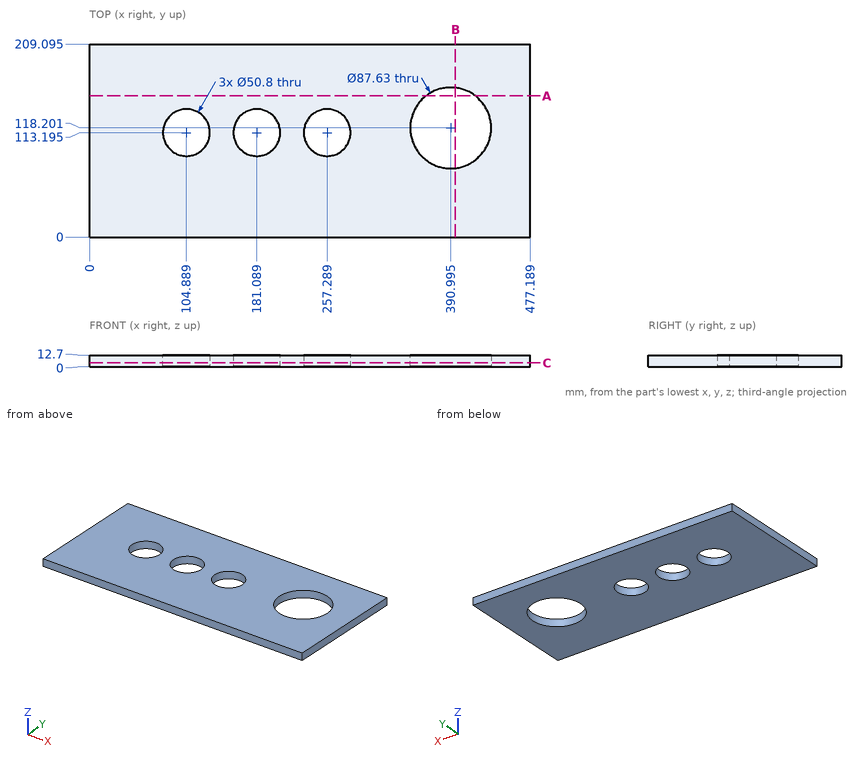
Geometry: see drawing. Coordinates: mm, zero at the bounding-box minimum. Round coordinates to 2 decimals unless told otherwise and drop trailing zeros. Loops run counter-clockwise (first coordinate to the right, second up) from the corner with the lowest first, then second, coordinate; pieces in that order, holes last. Notation, with made-up numbers: M 48.5,25 L 84.5,25 A19 cw 84.5,56 Z; hole C 24.25,58.5 d1. An arc over 180 degrees is marked long. Use a Markdown table: item, result. Add a question column.
1. Ray query, line 1 along X through (y, z) = (96.5, 4) (1 decimal); line 2 along Y through (x, z) = (429, 2.5) (1 decimal); line 3 along Y through (x, z) = (420, 3.5) (1 decimal). Return the intervals inside material, ascending. Write a range as [from, to].
2. Cut plane C-C, the plane z = 4.25. Output: boundary loops of the cut face in (x, y) (1 decimal), and give its area (3 significant figures).
3. Cut plane A-A, the plane y = 153. Output: boundary loops of the cut face in (x, z).
4. Cut plane B-B, the plane x = 396. Output: boundary loops of the cut face in (y, z) (1 decimal).
Solution:
| question | item | result |
|---|---|---|
| 1 | line 1 | x = [0, 85.7], [124, 161.9], [200.2, 238.1], [276.4, 352.9], [429.1, 477.2] |
| 1 | line 2 | y = [0, 96.4], [140, 209.1] |
| 1 | line 3 | y = [0, 85.4], [151, 209.1] |
| 2 | outline | M 0,0 L 477.2,0 L 477.2,209.1 L 0,209.1 Z; hole C 104.9,113.2 d50.8; hole C 181.1,113.2 d50.8; hole C 257.3,113.2 d50.8; hole C 391,118.2 d87.6 |
| 2 | area | 87,700 mm2 |
| 3 | outline | M 0,0 L 364.37,0 L 364.37,12.7 L 0,12.7 Z; M 417.62,0 L 477.19,0 L 477.19,12.7 L 417.62,12.7 Z |
| 4 | outline | M 0,0 L 74.7,0 L 74.7,12.7 L 0,12.7 Z; M 161.7,0 L 209.1,0 L 209.1,12.7 L 161.7,12.7 Z |
